Input: part model. Units: mm. Frame: model coordinates. Round coordinates to 2 decimals unless told otherwise and drop trailing zeros. Loops run counter-clockwise (first coordinate to the right, second up) from the corner with the lowest first, then second, coordinate; pieces in that order, holes last. Notation, with made-up numbers: (-8.5, 10) -> (24.5, 10) arc R19 cw to (24.5, 34) -> close; hole circle Ø3 at (-35.75, 29). An arc over 180 degrees is marked (long way). One line per question, with ' | ' between items. Start each with the question number.
Q1. Cut plane B-B on z = 106.25. Return loops of the section in (x, y).
Q2. Material intervals for L1, parallel to Z at x = -30, y = 1.45; L2, parallel to Z at x = -31, y = 0.3; L3, parallel to Z at x = 0.5, y = 0.15, sorted ascending.
Q3. Cut plane A-A on y = 1.15. State how many separate pieces and enclosed holes the cut face has, and give its area (3 significant figures).
Q4. Contact query for a flat-ended pin moving along its axis: P1, Ø2.5, axis at x = 30, z = 99.318, coming from the -Y side. Output: stop coordinate, or through.
Q5. Mould query, pull axis Z, two halves, no side actions, for faces 1 (the face through (-31.18, 1.01, 98.24)), 2 (the face through (33.836, 0.986, 101.391)), 3 (the face through (33.354, 1.014, 98.228)). Classes: pulls with the +Z half, pulls with the -Z half, needs draft (parallel to the pull), parting line crosses it, or undercut.
Q6. Cut plane C-C on x = 25.5. Return loops of the section in (y, z), and give its area (3 significant figures).
Autodesk Inventor part; units mm, degrees
ref_plane "YZ Plane" through (0, 0, 0) normal (1, 0, 0) x (0, 1, 0)
ref_plane "XZ Plane" through (0, 0, 0) normal (0, 1, 0) x (-1, 0, 0)
ref_plane "XY Plane" through (0, 0, 0) normal (0, 0, 1) x (1, 0, 0)
sketch "Sketch1" plane through (0, 0, 0) normal (0, 1, 0) x (-1, 0, 0)
  circle A0 centre (0, 0) radius 110 construction
  arc A1 (43.0581, -98.5) -> (-43.0581, -98.5) centre (0, 0) ccw
  line L0 (0, -107.5) -> (0, -98.5) construction
  line L1 (0, -98.5) -> (0, -73.5) construction
  line L2 (0, -98.5) -> (-43.0581, -98.5) construction
  line L3 (0, -98.5) -> (43.0581, -98.5) construction
  line L4 (43.0581, -98.5) -> (-43.0581, -98.5) construction
  line L5 (-18.0581, -73.5) -> (18.0581, -73.5)
  arc A2 (43.0581, -98.5) -> (18.0581, -73.5) centre (18.0581, -98.5) ccw
  arc A3 (-18.0581, -73.5) -> (-43.0581, -98.5) centre (-18.0581, -98.5) ccw
  line L6 (0, 107.5) -> (0, 97.5) construction
  line L7 (0, 97.5) -> (-22.5, 97.5) construction
  line L8 (-22.5, 97.5) -> (-22.5, 82.5) construction
  line L9 (22.5, 82.5) -> (22.5, 97.5) construction
  line L10 (22.5, 90) -> (-22.5, 90) construction
  line L11 (15, 97.5) -> (-15, 97.5)
  line L12 (-15, 82.5) -> (15, 82.5)
  arc A4 (15, 82.5) -> (15, 97.5) centre (15, 90) ccw
  arc A5 (-15, 97.5) -> (-15, 82.5) centre (-15, 90) ccw
  line L13 (22.5, 82.5) -> (17.5, 82.5) construction
  line L14 (17.5, 82.5) -> (17.5, 77.5) construction
  circle A6 centre (17.5, 77.5) radius 1.6
  circle A7 centre (-17.5, 77.5) radius 1.6
  line L15 (-58.3363, 79.5495) -> (-79.5495, 58.3363)
  arc A8 (-47.7297, 68.9429) -> (-58.3363, 79.5495) centre (-53.033, 74.2462) ccw
  arc A9 (-79.5495, 58.3363) -> (-68.9429, 47.7297) centre (-74.2462, 53.033) ccw
  line L16 (-68.9429, 47.7297) -> (-47.7297, 68.9429)
  circle A10 centre (-67.1751, 42.4264) radius 1.6
  circle A11 centre (-42.4264, 67.1751) radius 1.6
  line L17 (-97.5, 15) -> (-97.5, -15)
  arc A12 (-82.5, 15) -> (-97.5, 15) centre (-90, 15) ccw
  arc A13 (-97.5, -15) -> (-82.5, -15) centre (-90, -15) ccw
  line L18 (-82.5, -15) -> (-82.5, 15)
  circle A14 centre (-77.5, -17.5) radius 1.6
  circle A15 centre (-77.5, 17.5) radius 1.6
  line L19 (-79.5495, -58.3363) -> (-58.3363, -79.5495)
  arc A16 (-68.9429, -47.7297) -> (-79.5495, -58.3363) centre (-74.2462, -53.033) ccw
  arc A17 (-58.3363, -79.5495) -> (-47.7297, -68.9429) centre (-53.033, -74.2462) ccw
  line L20 (-47.7297, -68.9429) -> (-68.9429, -47.7297)
  circle A18 centre (-42.4264, -67.1751) radius 1.6
  circle A19 centre (-67.1751, -42.4264) radius 1.6
  line L21 (-15, -97.5) -> (15, -97.5)
  arc A20 (-15, -82.5) -> (-15, -97.5) centre (-15, -90) ccw
  arc A21 (15, -97.5) -> (15, -82.5) centre (15, -90) ccw
  line L22 (15, -82.5) -> (-15, -82.5)
  circle A22 centre (17.5, -77.5) radius 1.6
  circle A23 centre (-17.5, -77.5) radius 1.6
  line L23 (58.3363, -79.5495) -> (79.5495, -58.3363)
  arc A24 (47.7297, -68.9429) -> (58.3363, -79.5495) centre (53.033, -74.2462) ccw
  arc A25 (79.5495, -58.3363) -> (68.9429, -47.7297) centre (74.2462, -53.033) ccw
  line L24 (68.9429, -47.7297) -> (47.7297, -68.9429)
  circle A26 centre (67.1751, -42.4264) radius 1.6
  circle A27 centre (42.4264, -67.1751) radius 1.6
  line L25 (97.5, -15) -> (97.5, 15)
  arc A28 (82.5, -15) -> (97.5, -15) centre (90, -15) ccw
  arc A29 (97.5, 15) -> (82.5, 15) centre (90, 15) ccw
  line L26 (82.5, 15) -> (82.5, -15)
  circle A30 centre (77.5, 17.5) radius 1.6
  circle A31 centre (77.5, -17.5) radius 1.6
  line L27 (79.5495, 58.3363) -> (58.3363, 79.5495)
  arc A32 (68.9429, 47.7297) -> (79.5495, 58.3363) centre (74.2462, 53.033) ccw
  arc A33 (58.3363, 79.5495) -> (47.7297, 68.9429) centre (53.033, 74.2462) ccw
  line L28 (47.7297, 68.9429) -> (68.9429, 47.7297)
  circle A34 centre (42.4264, 67.1751) radius 1.6
  circle A35 centre (67.1751, 42.4264) radius 1.6
  line L29 (58.3363, -58.3363) -> (51.2652, -51.2652) construction
  line L30 (40.6586, -61.8718) -> (61.8718, -40.6586)
  arc A36 (40.6586, -61.8718) -> (44.5267, -89.5398) centre (53.033, -74.2462) ccw
  arc A37 (89.5398, -44.5267) -> (61.8718, -40.6586) centre (74.2462, -53.033) ccw
  line L31 (0, -73.5) -> (0, -66.5) construction
  arc A38 (44.5267, 89.5398) -> (40.6586, 61.8718) centre (53.033, 74.2462) ccw
  line L32 (61.8718, 40.6586) -> (40.6586, 61.8718)
  arc A39 (61.8718, 40.6586) -> (89.5398, 44.5267) centre (74.2462, 53.033) ccw
  arc A40 (-89.5398, 44.5267) -> (-61.8718, 40.6586) centre (-74.2462, 53.033) ccw
  line L33 (-40.6586, 61.8718) -> (-61.8718, 40.6586)
  arc A41 (-40.6586, 61.8718) -> (-44.5267, 89.5398) centre (-53.033, 74.2462) ccw
  arc A42 (-44.5267, -89.5398) -> (-40.6586, -61.8718) centre (-53.033, -74.2462) ccw
  line L34 (-61.8718, -40.6586) -> (-40.6586, -61.8718)
  arc A43 (-61.8718, -40.6586) -> (-89.5398, -44.5267) centre (-74.2462, -53.033) ccw
  arc A44 (89.5398, -44.5267) -> (89.5398, 44.5267) centre (0, 0) ccw
  arc A45 (44.5267, 89.5398) -> (-44.5267, 89.5398) centre (0, 0) ccw
  arc A46 (-89.5398, 44.5267) -> (-89.5398, -44.5267) centre (0, 0) ccw
  line L35 (43.0581, -98.5) -> (48.0581, -98.5) construction
  line L36 (48.0581, -98.5) -> (48.0581, -88.5) construction
  circle A47 centre (48.0581, -88.5) radius 1.6
  circle A48 centre (-48.0581, -88.5) radius 1.6
  line L37 (18.0581, -66.5) -> (-18.0581, -66.5)
  arc A49 (17.5, -66.5) -> (43.0581, -59.4724) centre (19.5145, -23.8377) ccw
  arc A50 (-44.5267, -58.0038) -> (-18.0581, -66.5) centre (-19.5089, -25.5422) ccw
  point P0 (0, 90)
  point P1 (-45.9619, 70.7107)
  point P2 (-82.5, 17.5)
  point P3 (-70.7107, -45.9619)
  point P4 (-17.5, -82.5)
  point P5 (45.9619, -70.7107)
  point P6 (82.5, -17.5)
  point P7 (70.7107, 45.9619)
  point P8 (35.7159, -76.7698)
  dimension "d0" = 220
  dimension "d1" = 215
  dimension "d2" = 9
  dimension "d3" = 25
  dimension "d4" = 10
  dimension "d5" = 22.5
  dimension "d6" = 15
  dimension "d7" = 45
  dimension "d8" = 5
  dimension "d9" = 5
  dimension "d10" = 3.2
  dimension "d15" = 86.1162
  dimension "d16" = 45
  dimension "d19" = 360
  dimension "d22" = 10
  dimension "d23" = 7
  dimension "d26" = 360
  dimension "d33" = 5
  dimension "d34" = 10
  dimension "d35" = 3.2
extrude "Extrusion1" add sketch "Sketch1" along normal blind 2 contours A2 L5 A3 A1
fillet "Fillet2" radius 2 6 edges at (-44.5267, 1, 89.5398) (44.5267, 1, 89.5398) (89.5398, 1, 44.5267) (89.5398, 1, -44.5267) (-89.5398, 1, -44.5267) (-89.5398, 1, 44.5267)
sketch "Sketch4" plane through (0, 2, 0) normal (0, 1, 0) x (1, 0, 0)
  circle A0 centre (0, 0) radius 103.75 construction
  line L0 (0, -103.75) -> (-30, -103.75) construction
  line L1 (-30, -103.75) -> (-30, -99.318) construction
  line L2 (0, -103.75) -> (0, -91.6543) construction
  line L3 (0, 0) -> (-10.2863, 0) construction
  circle A1 centre (-30, -99.318) radius 1.6
  circle A2 centre (30, -99.318) radius 1.6
  circle A3 centre (99.318, -30) radius 1.6
  circle A4 centre (99.318, 30) radius 1.6
  circle A5 centre (-99.318, -30) radius 1.6
  circle A6 centre (-99.318, 30) radius 1.6
  dimension "d45" = 207.5
  dimension "d46" = 30
  dimension "d47" = 3.2
  dimension "d50" = 90
extrude "Extrusion4" cut sketch "Sketch4" against normal blind 2
sketch "Sketch5" plane through (0, 2, 0) normal (0, 1, 0) x (1, 0, 0)
  circle A0 centre (0, 0) radius 100
  arc A1 (-41.3697, -91.0415) -> (41.3697, -91.0415) centre (0, 0) ccw
  circle A2 centre (0, 0) radius 107.5
  circle A3 centre (-30, -99.318) radius 1.6 construction
  circle A4 centre (-30, -99.318) radius 1.6 construction
  circle A5 centre (30, -99.318) radius 1.6 construction
  circle A6 centre (30, -99.318) radius 1.6 construction
  circle A7 centre (-22.8014, -101.2134) radius 1.6
  arc A8 (-30, -99.318) -> (-22.8014, -101.2134) centre (0, 0) ccw construction
  line L0 (-26.4177, -100.3303) -> (-25.4629, -96.7039) construction
  line L1 (-26.4177, -100.3303) -> (-24.1782, -100.92) construction
  line L2 (-26.4177, -100.3303) -> (-27.3726, -103.9567) construction
  line L3 (0, -100) -> (0, -107.5) construction
  arc A9 (-43.0581, 98.5) -> (43.0581, 98.5) centre (0, 0) ccw construction
  line L4 (-28.3384, -103.6976) -> (-26.4299, -96.4493)
  line L5 (-26.4299, -96.4493) -> (-24.4958, -96.9585) construction
  line L6 (-24.4958, -96.9585) -> (-26.4044, -104.2068)
  line L7 (-26.4055, -104.2113) -> (-28.3396, -103.7021) construction
  line L8 (-28.3396, -103.7021) -> (-24.4958, -96.9585) construction
  line L9 (-26.4299, -96.4493) -> (-26.4055, -104.2113) construction
  line L10 (-26.4299, -96.4493) -> (-26.4286, -96.4444)
  line L11 (-24.4958, -96.9585) -> (-24.4946, -96.9537)
  line L12 (28.3384, -103.6976) -> (26.4299, -96.4493)
  line L13 (24.4958, -96.9585) -> (26.4044, -104.2068)
  line L14 (26.4299, -96.4493) -> (26.4286, -96.4444)
  line L15 (24.4958, -96.9585) -> (24.4946, -96.9537)
  circle A10 centre (22.8014, -101.2134) radius 1.6
  arc A11 (-38.542, -96.3254) -> (-30, -99.318) centre (0, 0) ccw construction
  line L16 (0, 0) -> (-38.542, -96.3254) construction
  line L17 (0, 0) -> (-30, -99.318) construction
  line L18 (-34.3036, -97.9149) -> (-40.5197, -95.7371) construction
  line L19 (-34.3036, -97.9149) -> (-33.0637, -94.3758) construction
  line L20 (-34.3036, -97.9149) -> (-35.5435, -101.454) construction
  line L21 (-34.5982, -101.7802) -> (-32.12, -94.7064)
  line L22 (-34.0075, -94.0451) -> (-36.4857, -101.1189)
  line L23 (-34.5998, -101.7846) -> (-34.0075, -94.0451) construction
  line L24 (-32.12, -94.7064) -> (-36.4873, -101.1233) construction
  line L25 (-34.0075, -94.0451) -> (-34.0059, -94.0404)
  line L26 (-32.12, -94.7064) -> (-32.1183, -94.7017)
  line L27 (34.5982, -101.7802) -> (32.12, -94.7064)
  line L28 (34.0075, -94.0451) -> (36.4857, -101.1189)
  line L29 (34.0075, -94.0451) -> (34.0059, -94.0404)
  line L30 (32.12, -94.7064) -> (32.1183, -94.7017)
  dimension "d54" = 3.2
  dimension "d56" = 90
  dimension "d57" = 90
  dimension "d58" = 2
  dimension "d62" = 5
  dimension "d63" = 90
  dimension "d64" = 90
  dimension "d65" = 2
extrude "Extrusion6" cut sketch "Sketch5" against normal blind 10 contours A0 L26 L21 A2 L22 L25 | L29 L28 A2 L27 L30 A0
fillet "Fillet4" radius 2 4 edges at (34.5982, 1, 101.7802) (32.1183, 1, 94.7017) (-34.5982, 1, 101.7802) (-32.1183, 1, 94.7017)
sketch "Sketch6" plane through (0, 2, 0) normal (0, 1, 0) x (1, 0, 0)
  line L0 (-36.4857, -101.1189) -> (-34.0059, -94.0404)
  line L1 (-36.4857, -101.1189) -> (-34.0059, -94.0404)
  line L2 (-34.0059, -94.0404) -> (32.6146, -91.3584)
  arc A0 (34.0059, -94.0404) -> (41.3697, -91.0415) centre (0, 0) ccw
  line L3 (32.6146, -91.3584) -> (34.0059, -94.0404)
  line L4 (34.0059, -94.0404) -> (36.4857, -101.1189)
  line L5 (34.0059, -94.0404) -> (36.4857, -101.1189)
  line L6 (36.4857, -101.1189) -> (62.3564, -110.1825)
  line L7 (62.3564, -110.1825) -> (150.1312, 20.0804)
  line L8 (150.1312, 20.0804) -> (83.4633, 106.272)
  line L9 (83.4633, 106.272) -> (-86.1797, 106.272)
  line L10 (-86.1797, 106.272) -> (-127.6527, -26.6706)
  line L11 (-127.6527, -26.6706) -> (-61.5058, -119.0367)
  line L12 (-61.5058, -119.0367) -> (-36.4857, -101.1189)
extrude "Extrusion7" cut sketch "Sketch6" against normal blind 10
properties part number "MettalringUnten_v3"
Results:
1) outline: (-16.35, 0) -> (16.35, 0) -> (16.35, 2) -> (-16.35, 2) -> close
2) L1: 95.39 to 97.72, 100.92 to 103.23 | L2: 95.22 to 98.07, 100.57 to 102.93 | L3: 100 to 107.5
3) separate pieces: 1 | enclosed holes: 2 | area: 490 mm^2
4) P1: through
5) face 1: undercut | face 2: parting line crosses it | face 3: pulls with the -Z half
6) outline: (0, 96.69) -> (2, 96.69) -> (2, 104.43) -> (0, 104.43) -> close | area: 15.5 mm^2
